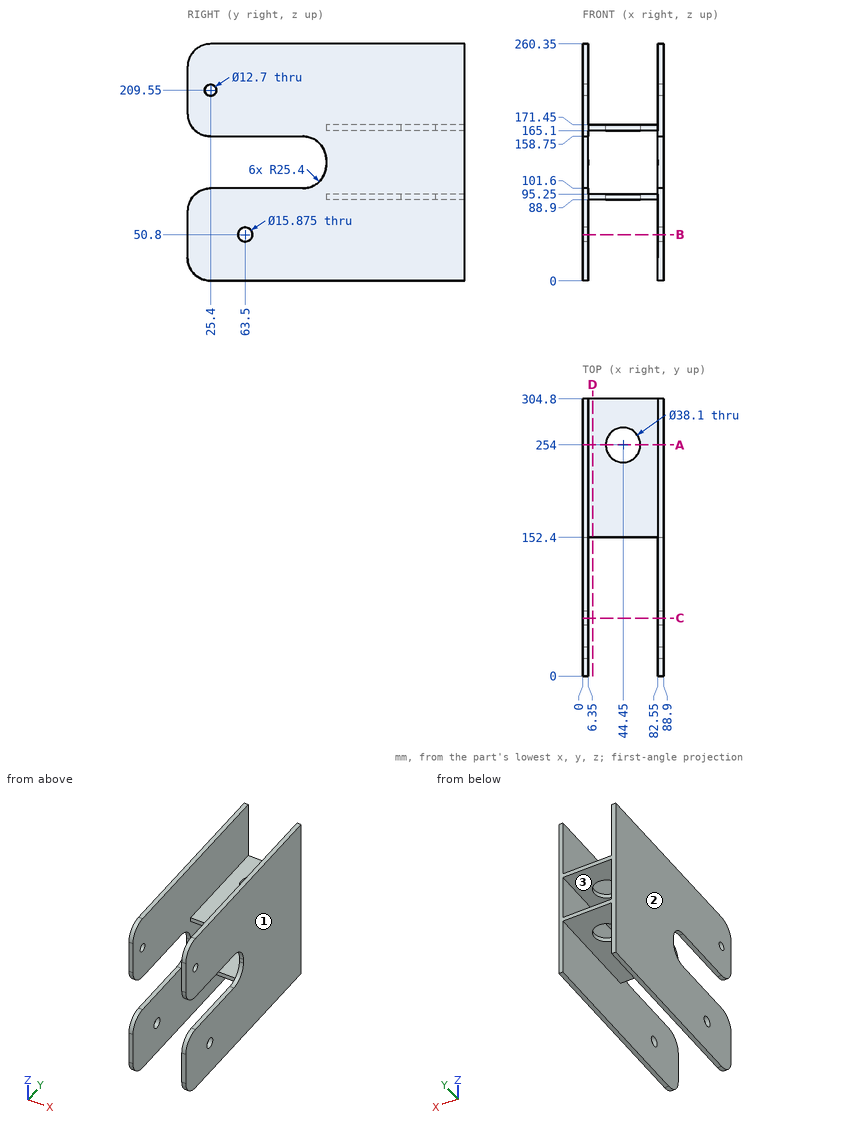
Geometry: see drawing. Coordinates: mm, zero at the bounding-box minimum. Coordinates: 2 decimals unless noted, no trailing zeros. Loops run counter-clockwise (first coordinate to the right, second up) from the corner with the lowest first, then second, coordinate; pieces in that order, holes last.
Q1. Draft query along X for the marked faces 1, 2 and 3. Return one class per face: +X half, -X half, draft (parallel to the pull), parting line (faces both ways), or undercut.
Q2. Cut plane B-B (z = 50.8). Output: boundary loops of the cut face in (x, y), then the cut area to 3 significant figures.
Q3. Cut plane D-D (x = 11). Output: boundary loops of the cut face in (y, z).
Q4. Contact query for flat-ended pins moving along their axis: pin 1 (12 mm diameter, centred on x = 47, y = 153.5, fed in from -Z); pin 2 (7 mm diameter, centred on x = 86.5, z = 129, fed in from -Y); pin 3 (9.5 mm diameter, centred on y = 63.5, z = 50.8, fed in from -X). Output: stop coordinate, or through.
Q5. Material intervals for line 1 (Z direction, x = 85, y = 25); line 2 (Z direction, x = 2, y = 63.5); line 3 (Y direction, x = 4.5, z = 209.55), sorted ascending.
Q6. Cut plane C-C (y = 63.5). Output: boundary loops of the cut face in (x, z), then the cut area to 3 significant figures.
Q7. Cut plane A-A (y = 254). Output: boundary loops of the cut face in (x, z), then the cut area to 3 significant figures.
Working result:
1. face 1: +X half
1. face 2: -X half
1. face 3: undercut
2. outline: (0, 0) - (6.35, 0) - (6.35, 55.56) - (0, 55.56) - close; (0, 71.44) - (6.35, 71.44) - (6.35, 304.8) - (0, 304.8) - close; (82.55, 0) - (88.9, 0) - (88.9, 55.56) - (82.55, 55.56) - close; (82.55, 71.44) - (88.9, 71.44) - (88.9, 304.8) - (82.55, 304.8) - close
2. area: 3,670 mm2
3. outline: (152.4, 88.9) - (304.8, 88.9) - (304.8, 95.25) - (152.4, 95.25) - close; (152.4, 165.1) - (304.8, 165.1) - (304.8, 171.45) - (152.4, 171.45) - close
4. pin 1: stops at z = 88.9
4. pin 2: stops at y = 152.36
4. pin 3: passes through
5. line 1: z = 0 to 101.6, 158.75 to 203.21, 215.89 to 260.35
5. line 2: z = 0 to 42.86, 58.74 to 101.6, 158.75 to 260.35
5. line 3: y = 0 to 19.05, 31.75 to 304.8
6. outline: (0, 0) - (6.35, 0) - (6.35, 42.86) - (0, 42.86) - close; (0, 58.74) - (6.35, 58.74) - (6.35, 101.6) - (0, 101.6) - close; (0, 158.75) - (6.35, 158.75) - (6.35, 260.35) - (0, 260.35) - close; (82.55, 0) - (88.9, 0) - (88.9, 42.86) - (82.55, 42.86) - close; (82.55, 58.74) - (88.9, 58.74) - (88.9, 101.6) - (82.55, 101.6) - close; (82.55, 158.75) - (88.9, 158.75) - (88.9, 260.35) - (82.55, 260.35) - close
6. area: 2,380 mm2
7. outline: (0, 0) - (6.35, 0) - (6.35, 88.9) - (25.4, 88.9) - (25.4, 95.25) - (6.35, 95.25) - (6.35, 165.1) - (25.4, 165.1) - (25.4, 171.45) - (6.35, 171.45) - (6.35, 260.35) - (0, 260.35) - close; (63.5, 88.9) - (82.55, 88.9) - (82.55, 0) - (88.9, 0) - (88.9, 260.35) - (82.55, 260.35) - (82.55, 171.45) - (63.5, 171.45) - (63.5, 165.1) - (82.55, 165.1) - (82.55, 95.25) - (63.5, 95.25) - close
7. area: 3,790 mm2
